Work out the finished part from the listing and answer in its coordinate system (mm). A direction names the side the tool comes from. Round coordinates to 2 decimals unless told otherwise and drop trailing zeros. Order: outer loops, then holes, each group sorted by start corner. A loop starts at its lowest first (then second) coordinate and runs counter-clockwise, first axis right, second up. Notation, with made-up numbers: (20.25, 49.5) -> (62.25, 49.5) arc R28 ccw to (62.25, 73.5) -> close; hole circle Ø10 at (-12.5, 32). An arc over 180 degrees is marked (long way). Use one line per item in the form item = value.
```python
from build123d import *

# Parameters (mm, degrees)
CROQUIS1_R              = 2
SALIENTE_EXTRUIR1_DEPTH = 8
CROQUIS2_R              = 3
CORTAR_EXTRUIR1_DEPTH   = 9


with BuildPart() as part:
    # Croquis1 → Saliente-Extruir1 (new body)
    with BuildSketch(Plane(origin=(0, 0, 0), x_dir=(1, 0, 0), z_dir=(0, 1, 0))):
        with BuildLine():
            Line((25, 0), (38, 0))
            Line((38, 0), (38, 15))
            ThreePointArc((38, 15), (35.071067812, 22.071067812), (28, 25))
            Line((28, 25), (0, 25))
            ThreePointArc((0, 25), (-3.535533906, 23.535533906), (-5, 20))
            Line((-5, 20), (-5, 0))
            Line((-5, 0), (0, 0))
            Line((0, 0), (0, 20))
            Line((0, 20), (25, 20))
            Line((25, 20), (25, 0))
        make_face()
        with Locations(Location((32.5, 8, 0), (0, 0, 270))):
            Circle(CROQUIS1_R, mode=Mode.SUBTRACT)
    extrude(amount=SALIENTE_EXTRUIR1_DEPTH)

    # Croquis2 → Cortar-Extruir1 (cut)
    with BuildSketch(Plane.XZ):
        with Locations(Location((32.5, -8, 0), (0, 0, 270))):
            Circle(CROQUIS2_R)
    extrude(amount=-CORTAR_EXTRUIR1_DEPTH, mode=Mode.SUBTRACT)


solid = part.part
```
Item 1: Determine the mould class of faces 1 (the flat face through (0, 4, -10)), 2 (the flat face through (12, 4, -20)), 3 (the cylindrical face through (35.03, 3.94, -9.61)) for opening direction Z: released by +Z, released by -Z, zero draft, split by the parting line, or undercut.
Findings:
face_1 = zero draft
face_2 = released by +Z
face_3 = undercut
Item 2: The part is cut by section D-D, the plane x = 13.5. Give the vertices of the cut face in (y, z), and give its area (3 significant figures).
Findings:
outline = (0, -25) -> (8, -25) -> (8, -20) -> (0, -20) -> close
area = 40.0 mm^2
Item 3: For faces 4 (the flat face through (14, 4, -25)), 5 (the flat face through (25, 4, -10)), determine the directions among +Z, -Z, +X, -X, +Y, -Y from which every point of the face is accessible in a straight line to the end or side of a thin tool.
Findings:
face_4 = -Z, +X, -X, +Y, -Y
face_5 = +Z, +Y, -Y
Item 4: The part is cut by section A-A, the plane z = -8. Give the vertices of the cut face in (x, y), and give its area (3 significant figures).
Findings:
outline = (-5, 0) -> (0, 0) -> (0, 8) -> (-5, 8) -> close; (25, 0) -> (29.5, 0) -> (29.5, 8) -> (25, 8) -> close; (35.5, 0) -> (38, 0) -> (38, 8) -> (35.5, 8) -> close
area = 96.0 mm^2
Item 5: Consider line 1 along X through (y, z) = (3.5, -8); line 2 along X through (y, z) = (6.25, -5.75); line 3 along X through (y, z) = (2, -15). Determine where each line is inside the solid, lowest interval first.
Findings:
line_1 = -5 to 0, 25 to 29.5, 35.5 to 38
line_2 = -5 to 0, 25 to 30.52, 34.48 to 38
line_3 = -5 to 0, 25 to 38
Item 6: Flat-ended cylindrical pins translate along their axes: P1, Ø2, axis at y = 4, z = -18, coming from the +X side; P2, Ø3, axis at x = 7.5, y = 3, coming from the +Z side; P3, Ø1, axis at x = 1.5, z = -8, coming from the -Y side; P4, Ø1.5, axis at x = 33.5, y = 6.5, coming from the -Z side. Find the tip coordinate at first contact, or state that the pin passes through.
Findings:
P1 = 37.8
P2 = -20
P3 = through
P4 = -23.8
Item 7: The part is cut by section C-C, the plane x = 32.5. Give the vertices of the cut face in (y, z), and give its area (3 significant figures).
Findings:
outline = (0, -23.93) -> (8, -23.93) -> (8, -11) -> (0, -11) -> close; (0, -5) -> (8, -5) -> (8, 0) -> (0, 0) -> close
area = 143 mm^2
Item 8: The part is cut by section B-B, the plane y = 5.75. Give the vertices of the cut face in (x, z).
Findings:
outline = (-5, -20) arc R5 ccw to (0, -25) -> (28, -25) arc R10 ccw to (38, -15) -> (38, 0) -> (25, 0) -> (25, -20) -> (0, -20) -> (0, 0) -> (-5, 0) -> close; hole circle Ø6 at (32.5, -8)
